Geometry: final body of the model. Coordinates: model frame, mm. Face numbers are marked on the shaded views. A direction names the side the tool comes from. Round coordinates to 2 decimals unless told otherwise and drop trailing zeros. Loops run counter-clockwise (first coordinate to the right, second up) from the corner with the lowest first, then second, coordinate; pieces in that order, holes last. Notation, with made-up numbers: M 8,39.5 L 28,39.5 A20 ccw 28,71.5 Z; hole C 38.25,-3 d3. An arc over 180 degrees is marked long. Return JSON: item names as keys, results as strings.
from build123d import *

# Parameters (mm, degrees)
SKETCH1_R               = 1.75
BOSS_EXTRUDE1_DEPTH     = 4
SKETCH2_R               = 2.15
CUT_EXTRUDE1_DEPTH      = 5
BOSS_EXTRUDE5_START     = -1.8499999
BOSS_EXTRUDE5_OUTLINE_R = 2
BOSS_EXTRUDE5_DEPTH     = 11.8499999
BOSS_EXTRUDE5_START_2   = -3
BOSS_EXTRUDE5_2_DEPTH   = 7.824935333
SKETCH3_R               = 2.15
CUT_EXTRUDE2_DEPTH      = 5
BOSS_EXTRUDE2_START     = 4
SKETCH4_W               = 8
SKETCH4_H               = 7.3
SKETCH4_R               = 2.15
BOSS_EXTRUDE2_DEPTH     = 4
BOSS_EXTRUDE3_START     = 4
SKETCH5_W               = 8
SKETCH5_H               = 7.3
SKETCH5_R               = 2.15
BOSS_EXTRUDE3_DEPTH     = 4
SKETCH6_R               = 0.4895
BOSS_EXTRUDE4_DEPTH     = 10
FILLET1_R               = 2


with BuildPart() as part:
    # Sketch1 → Boss-Extrude1 (new, symmetric)
    with BuildSketch(Plane(origin=(0, 0, 0), x_dir=(0, 0, -1), z_dir=(1, 0, 0))):
        with BuildLine():
            Line((-3.65, 4.824935233), (3.65, 4.824935233))
            ThreePointArc((3.65, 4.824935233), (4.277996026, 4.277996026), (4.824935233, 3.65))
            Line((4.824935233, 3.65), (4.824935233, -3.65))
            ThreePointArc((4.824935233, -3.65), (-4.277996026, -4.277996026), (-3.65, 4.824935233))
        make_face()
        Circle(SKETCH1_R, mode=Mode.SUBTRACT)
    extrude(amount=BOSS_EXTRUDE1_DEPTH, both=True)

    # Sketch2 → Cut-Extrude1 (cut)
    with BuildSketch(Plane(origin=(0, 4.824935233, 0), x_dir=(1, 0, 0), z_dir=(0, 1, 0))):
        with Locations(Location((0, 0, 0), (0, 0, 270))):
            Circle(SKETCH2_R)
    extrude(amount=-CUT_EXTRUDE1_DEPTH, mode=Mode.SUBTRACT)

    # Boss-Extrude5: read off the stored shape, not the designer's step
    # Boss-Extrude5 outline → Boss-Extrude5 (add)
    with BuildSketch(Plane(origin=(4, 0, 0), x_dir=(0, 0, -1), z_dir=(1, 0, 0)).offset(BOSS_EXTRUDE5_START)):
        Circle(BOSS_EXTRUDE5_OUTLINE_R)
    extrude(amount=BOSS_EXTRUDE5_DEPTH)

    # Boss-Extrude5 2 outline → Boss-Extrude5 2 (add)
    with BuildSketch(Plane(origin=(0, 0, 0), x_dir=(1, 0, 0), z_dir=(0, 1, 0)).offset(BOSS_EXTRUDE5_START_2)):
        with BuildLine():
            Line((2.1500001, -3), (2.15, 0))
            ThreePointArc((2.15, 0), (1.52027958, -1.52027958), (0, -2.15))
            Line((0, -2.15), (0, -3))
            Line((0, -3), (2.1500001, -3))
        make_face()
        with BuildLine():
            ThreePointArc((0, 2.15), (1.52027958, 1.52027958), (2.15, 0))
            Line((2.15, 0), (2.1500001, 3))
            Line((2.1500001, 3), (0, 3))
            Line((0, 3), (0, 2.15))
        make_face()
    extrude(amount=BOSS_EXTRUDE5_2_DEPTH)

    # Sketch3 → Cut-Extrude2 (cut)
    with BuildSketch(Plane(origin=(0, 0, -4.824935233), x_dir=(-1, 0, 0), z_dir=(0, 0, -1))):
        Circle(SKETCH3_R)
    extrude(amount=-CUT_EXTRUDE2_DEPTH, mode=Mode.SUBTRACT)

    # Sketch4 → Boss-Extrude2 (add)
    with BuildSketch(Plane(origin=(0, 4.824935233, 0), x_dir=(1, 0, 0), z_dir=(0, 1, 0)).offset(BOSS_EXTRUDE2_START)):
        Rectangle(SKETCH4_W, SKETCH4_H)
        with Locations(Location((0, 0, 0), (0, 0, 270))):
            Circle(SKETCH4_R, mode=Mode.SUBTRACT)
    extrude(amount=-BOSS_EXTRUDE2_DEPTH)

    # Sketch5 → Boss-Extrude3 (add)
    with BuildSketch(Plane(origin=(0, 0, -4.824935233), x_dir=(-1, 0, 0), z_dir=(0, 0, -1)).offset(BOSS_EXTRUDE3_START)):
        Rectangle(SKETCH5_W, SKETCH5_H)
        Circle(SKETCH5_R, mode=Mode.SUBTRACT)
    extrude(amount=-BOSS_EXTRUDE3_DEPTH)

    # Sketch6 → Boss-Extrude4 (add)
    with BuildSketch(Plane.XY.offset(3.65)):
        with BuildLine():
            Line((-2, 5.1645), (-5, 5.1645))
            ThreePointArc((-5, 5.1645), (-6.9895, 3.175), (-5, 1.1855))
            Line((-5, 1.1855), (-2, 1.1855))
            ThreePointArc((-2, 1.1855), (-0.0105, 3.175), (-2, 5.1645))
        make_face()
        with Locations((-5, 3.175)):
            Circle(SKETCH6_R, mode=Mode.SUBTRACT)
    extrude(amount=BOSS_EXTRUDE4_DEPTH)

    # Fillet1
    # the kernel refuses this fillet: 2 mm, written as the material it adds along each edge
    with BuildSketch(Plane(origin=(-2, 3.175, 3.65), x_dir=(0.03534330894551541, -0.9993752300876693, 0), z_dir=(-0.9993752300876693, -0.03534330894551541, 0))) as fillet1_piece_1:
        with BuildLine():
            CenterArc((1.9895 + FILLET1_R, FILLET1_R), FILLET1_R, 180, 90)
            Line((1.9895 + FILLET1_R, 0), (1.9895, 0))
            Line((1.9895, 0), (1.9895, FILLET1_R))
        make_face()
    revolve(axis=Axis((-2, 3.175, 3.65), (0, 0, 1)), revolution_arc=177.974555734)
    with BuildSketch(Plane(origin=(-2, 5.1645, 3.65), x_dir=(0, 0, 1), z_dir=(-1, 0, 0))) as fillet1_piece_2:
        with BuildLine():
            CenterArc((FILLET1_R, FILLET1_R), FILLET1_R, 180, 90)
            Line((0, FILLET1_R), (0, 0))
            Line((0, 0), (FILLET1_R, 0))
        make_face()
    extrude(amount=2)


solid = part.part
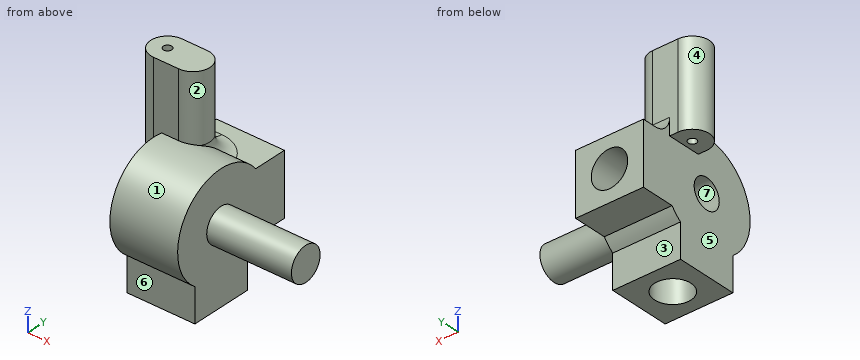
Q1. Pin query (flat end, axial travel): pin 1 (8 mm diameter, centred on x = 7.5, z = -5, fed in from -Y); pin 2 (0.9 mm diameter, centred on x = -6, y = 2.5, fed in from -Z); pin 3 (5.5 mm diameter, centred on x = 0, y = 0, fed in from -Z); pin 4 (5 mm diameter, centred on x = 7.5, y = -1, fed in from +Z). Return the tip coordinate at first contact, or that it passes through.
Determined:
{"pin 1": "stops at y = -5.22", "pin 2": "stops at z = 3.65", "pin 3": "stops at z = -8.82", "pin 4": "stops at z = 2"}
Q2. Material intervals for L1, parallel to Y at x = -5, z = 10.5; L2, parallel to X at y = 6, z = 0; L3, parallel to Y at x = -2.5, z = 0, sorted ascending.
Determined:
{"L1": "y = 1.19 to 2.69, 3.66 to 5.16", "L2": "x = -4 to -2.15, 2.15 to 4", "L3": "y = -6.05 to -1.75, 1.75 to 8.82"}
Q3. Section query D-D (y = -2.5). Output: boundary loops of the cut face in (x, z).
Determined:
{"outline": "M -4,-8.82 L 4,-8.82 L 4,5.51 L -4,5.51 Z"}
Q4. Section query A-A (z = -0.5). Output: boundary loops of the cut face in (x, y).
Determined:
{"outline": "M -4,-6.03 L 4,-6.03 L 4,-1.94 L 14,-1.94 L 14,1.94 L 4,1.94 L 4,8.82 L 2.09,8.82 L 2.09,0.5 A2.15 cw 2.09,-0.5 L 2.09,-1.68 L 1.35,-1.68 A2.15 cw -1.35,-1.68 L -4,-1.68 Z; M -4,1.68 L -2.09,1.68 L -2.09,8.82 L -4,8.82 Z"}
Q5. Section query C-C (y = -4.25). Output: boundary loops of the cut face in (x, z).
Determined:
{"outline": "M -4,-4.31 L 4,-4.31 L 4,4.31 L -4,4.31 Z"}
Q6. Section query B-B (x = 11.75). Output: boundary loops of the cut face in (y, z), plus the area to 3 significant figures.
Determined:
{"outline": "C 0,0 d4", "area": "12.6 mm^2"}
Q7. Reachability of the marked faces 1, 2 and 3 from +Z, -Z, +X, -X, +Y, -Y: full face, straight path, thin tool, end or side. Return the list, or none.
Determined:
{"face 1": "+X", "face 2": "+Z, +X", "face 3": "-Z, +X, -X, +Y"}
Q8. Pull-direction query (Y, two-part tool) for the marked faces 4, 5, 6 and 7; classes: pulls with the +Y half, pulls with the -Y half, needs draft (parallel to the pull), parting line crosses it, or undercut.
Determined:
{"face 4": "parting line crosses it", "face 5": "needs draft", "face 6": "pulls with the -Y half", "face 7": "undercut"}
